Geometry: final body of the model. Coordinates: model frame, mm. Face numbers are marked on the shaded views. A direction names the side the tool comes from. Round coordinates to 2 decimals unless told otherwise and drop trailing zeros. Loops run counter-clockwise (first coordinate to the right, second up) from the corner with the lowest first, then second, coordinate; pieces in that order, holes last. Notation, with made-up numbers: (11.5, 31) - (62.5, 31) arc R18 ccw to (62.5, 52) - close; hole circle Ø4 at (27.25, -24.5). An arc over 180 degrees is marked (long way). Return JSON: item names as keys, results as strings. Group by question number.
1. Section A-A on z = 0.25. Return loops of the section in (x, y), and give its area (3 significant figures).
2. Section B-B on z = -3.25. Return loops of the section in (x, y), and give its area (3 significant figures).
3. Draft query along X for the marked faces 3, 4 and 5. Return one class per face: +X half, -X half, draft (parallel to the pull), parting line (faces both ways), or undercut.
4. Set-up query: the marked faces 1 and 2. Return all of +Z, -Z, +X, -X, +Y, -Y with unobstructed straight access to the full face (end or side cutting, diameter ignored); none if empty.
5. First-contact query: pin 1 Ø6 at (x, z) = (3.5, 0) entering from +Y; pin 2 Ø3 at (x, y) = (-4, -4.5) entering from -Z; pin 3 Ø6 at (x, y) = (-2, 3) entering from -Z; pin 4 Ø1 at (x, z) = (-4, 7) entering from -Y. Flat tips, straight axial feed; report the tip coordinate or a pass-through.
6. Material intervals for probe 1 along Z at (x, y) = (2, -3); probe 2 along Y at (x, z) = (2.25, 0.25); probe 3 along X at (y, z) = (-5.25, 4.25), sorted ascending.
from build123d import *


with BuildPart() as part:
    # Sketch1 → Revolve1 (revolve)
    with BuildSketch(Plane(origin=(0, 0, 0), x_dir=(0, 0, -1), z_dir=(1, 0, 0))):
        with BuildLine():
            Line((-9.5, 1.2), (-9.5, 4.274328321))
            ThreePointArc((-9.5, 4.274328321), (-9.468228076, 4.367925391), (-9.386043428, 4.422839417))
            Line((-9.386043428, 4.422839417), (-3.5, 6))
            Line((-3.5, 6), (0.34625, 6))
            ThreePointArc((0.34625, 6), (0.454967668, 5.954967668), (0.5, 5.84625))
            Line((0.5, 5.84625), (0.5, 3.46125))
            ThreePointArc((0.5, 3.46125), (0.391282332, 3.416217668), (0.34625, 3.3075))
            Line((0.34625, 3.3075), (0.34625, 3))
            ThreePointArc((0.34625, 3), (0.391282332, 2.891282332), (0.5, 2.84625))
            Line((0.5, 2.84625), (1.26875, 2.84625))
            Line((1.26875, 2.84625), (1.4225, 3))
            Line((1.4225, 3), (7.9625, 3))
            Line((7.9625, 3), (9.386043428, 2.618562688))
            ThreePointArc((9.386043428, 2.618562688), (9.468228076, 2.563648662), (9.5, 2.470051592))
            Line((9.5, 2.470051592), (9.5, 0))
            Line((9.5, 0), (-9.002943725, 0))
            Line((-9.002943725, 0), (-9.5, 1.2))
        make_face()
    revolve(axis=Axis((0, 0, -9.5), (0, 0, 1)))


solid = part.part
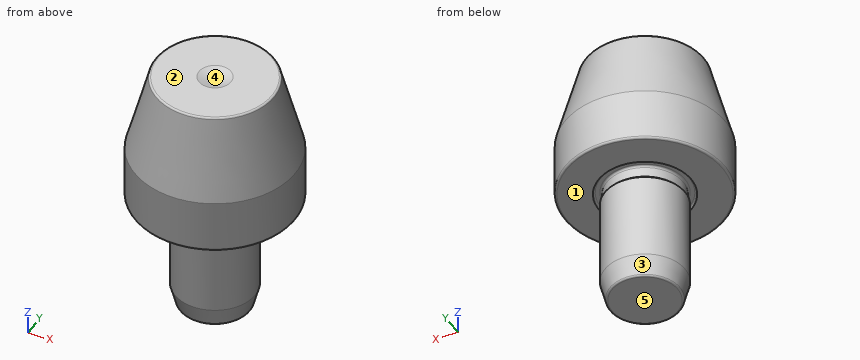
Taken from the geometry:
{
 "1": {"outline": "circle Ø12 at (0, 0)", "area": "113 mm2"},
 "2": {"outline": "circle Ø6 at (0, 0)", "area": "28.3 mm2"},
 "3": {"face 3": "parting line", "face 4": "undercut", "face 5": "draft"},
 "4": {"face 1": "-Z", "face 2": "+Z, +X, -X, +Y, -Y"},
 "5": {"pin 1": "y = 5.98", "pin 2": "z = -0.5", "pin 3": "z = -9.5", "pin 4": "y = -3.69"},
 "6": {"probe 1": "-0.5 to 9.5", "probe 2": "-5.56 to 5.56", "probe 3": "-2.46 to 2.46"}
}
